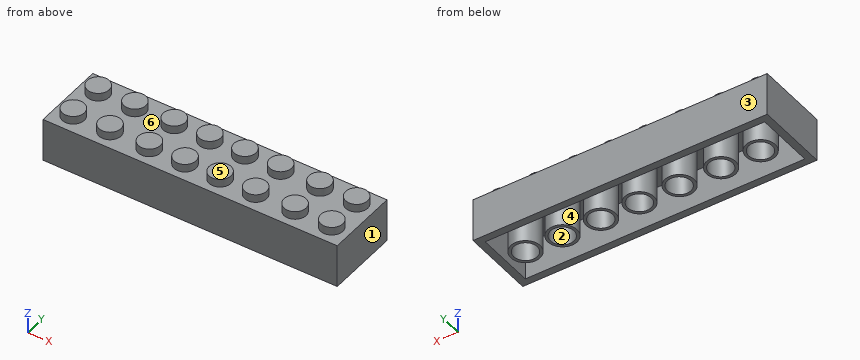
from build123d import *

# Parameters (mm, degrees)
F0_W     = 64.1604
F0_H     = 15.9258
F1_DEPTH = 9.4488
F2_R     = 2.4003
F3_DEPTH = 1.7526
F4_W     = 60.9346
F4_H     = 12.8524
F5_DEPTH = 8.128
F6_R     = 3.175
F7_DEPTH = 8.128
F8_R     = 2.5654
F9_DEPTH = 8.128


with BuildPart() as f1:
    # F0 (on Top) → F1 (new body)
    with BuildSketch(Plane.XY):
        Rectangle(F0_W, F0_H)
    extrude(amount=F1_DEPTH)

    # F2 (on face) → F3 (join)
    with BuildSketch(Plane.XY.offset(9.4488)):
        with Locations((-28.1813, -3.9878)):
            Circle(F2_R)
        with Locations((-20.1803, -3.9878)):
            Circle(F2_R)
        with Locations((-11.5951, -3.9878)):
            Circle(F2_R)
        with Locations((-3.8227, -3.9878)):
            Circle(F2_R)
        with Locations((3.8227, -3.9878)):
            Circle(F2_R)
        with Locations((11.5951, -3.9878)):
            Circle(F2_R)
        with Locations((20.1803, -3.9878)):
            Circle(F2_R)
        with Locations((28.1813, -3.9878)):
            Circle(F2_R)
        with Locations((28.1813, 3.9878)):
            Circle(F2_R)
        with Locations((20.1803, 3.9878)):
            Circle(F2_R)
        with Locations((11.5951, 3.9878)):
            Circle(F2_R)
        with Locations((3.8227, 3.9878)):
            Circle(F2_R)
        with Locations((-3.8227, 3.9878)):
            Circle(F2_R)
        with Locations((-11.5951, 3.9878)):
            Circle(F2_R)
        with Locations((-20.1803, 3.9878)):
            Circle(F2_R)
        with Locations((-28.1813, 3.9878)):
            Circle(F2_R)
    extrude(amount=F3_DEPTH)

    # F4 (on face) → F5 (cut)
    with BuildSketch(Plane(origin=(0, 0, 0), x_dir=(1, 0, 0), z_dir=(0, 0, -1))):
        Rectangle(F4_W, F4_H)
    extrude(amount=-F5_DEPTH, mode=Mode.SUBTRACT)

    # F6 (on face) → F7 (join)
    with BuildSketch(Plane(origin=(0, 0, 8.128), x_dir=(1, 0, 0), z_dir=(0, 0, -1))):
        with Locations((-25.222215, 0)):
            Circle(F6_R)
        with Locations((-16.592832, 0)):
            Circle(F6_R)
        with Locations((-7.534514, 0)):
            Circle(F6_R)
        with Locations((1.221147, 0)):
            Circle(F6_R)
        with Locations((9.622647, 0)):
            Circle(F6_R)
        with Locations((17.994031, 0)):
            Circle(F6_R)
        with Locations((26.055757, 0)):
            Circle(F6_R)
    extrude(amount=F7_DEPTH)

    # F8 (on face) → F9 (cut)
    with BuildSketch(Plane(origin=(0, 0, 0), x_dir=(1, 0, 0), z_dir=(0, 0, -1))):
        with Locations((-25.179168, 0)):
            Circle(F8_R)
        with Locations((-16.512433, 0)):
            Circle(F8_R)
        with Locations((-7.449481, 0)):
            Circle(F8_R)
        with Locations((1.221147, 0)):
            Circle(F8_R)
        with Locations((9.641448, 0)):
            Circle(F8_R)
        with Locations((18.037833, 0)):
            Circle(F8_R)
        with Locations((26.063653, 0)):
            Circle(F8_R)
    extrude(amount=-F9_DEPTH, mode=Mode.SUBTRACT)


solid = f1.part
Here's how the part is built. I have some questions about the finished solid (model axes, mm). Face numbers are marked on the shaded views. A direction names the side the tool comes from. Round coordinates to 2 decimals unless told otherwise and drop trailing zeros. Loops run counter-clockwise (first coordinate to the right, second up) from the corner with the lowest first, then second, coordinate; pieces in that order, holes last. Notation, with made-up numbers: (4, -7.75) -> (18, -7.75) arc R5 ccw to (18, 1.25) -> close; hole circle Ø11 at (70.25, 32.5). An arc over 180 degrees is marked (long way). Write each question's results on one line, items separated by ' | '.
(1) If we section it at A-A, the plane z = 7: Give the number of separate pieces and of enclosed holes in the cut face, then the cut area to 3 significant figures.
Worked answers:
separate pieces: 8 | enclosed holes: 8 | area: 316 mm2
(2) We'd pull the mould along X, two halves only. Please class the marked faces 1, 2 and 3: released by +X, released by -X, zero draft, split by the parting line, or undercut.
Worked answers:
face 1: released by +X | face 2: undercut | face 3: zero draft
(3) For the marked faces 4, 5 and 6, which set-ups out of +Z, -Z, +X, -X, +Y, -Y let a thin tool reach every point of the face, with its end or its side?
Worked answers:
face 4: -Z | face 5: +Z, +X, -X, +Y, -Y | face 6: +Z
(4) If we section it at C-C, the plane x = -27: List the corners of the cut face in (y, z) for me.
Worked answers:
outline: (-7.96, 0) -> (-6.43, 0) -> (-6.43, 8.13) -> (-2.63, 8.13) -> (-2.63, 0) -> (-1.81, 0) -> (-1.81, 8.13) -> (1.81, 8.13) -> (1.81, 0) -> (2.63, 0) -> (2.63, 8.13) -> (6.43, 8.13) -> (6.43, 0) -> (7.96, 0) -> (7.96, 9.45) -> (6.08, 9.45) -> (6.08, 11.2) -> (1.9, 11.2) -> (1.9, 9.45) -> (-1.9, 9.45) -> (-1.9, 11.2) -> (-6.08, 11.2) -> (-6.08, 9.45) -> (-7.96, 9.45) -> close
(5) If I drill on L1, parallel to X at y = 4.75, z = 7; L2, parallel to Y at x = -12, z = 3.75; L3, parallel to Y at x = 7.5, z = 6, over which ranges is the centre line in solid material (lowest first)?
Worked answers:
L1: -32.08 to -30.47, 30.47 to 32.08 | L2: -7.96 to -6.43, 6.43 to 7.96 | L3: -7.96 to -6.43, -2.36 to -1.41, 1.41 to 2.36, 6.43 to 7.96
(6) For P1, Ø3, axis at x = 1.22, y = 0, coming from the -Z side, with a flat end and sliding along its axis, tell me the tip position at first contact or that it passes through.
Worked answers:
P1: z = 8.13
